from build123d import *

# Parameters (mm, degrees)
SKETCH1_R                      = 46
SKETCH1_R_2                    = 36.05
SKETCH1_R_3                    = 30
BOSS_EXTRUDE1_DEPTH            = 2
BOSS_EXTRUDE2_START            = -2
SKETCH1_3_R                    = 46
SKETCH1_3_R_2                  = 36.05
BOSS_EXTRUDE2_DEPTH            = 8
CBORE_FOR_M3_SHCS2_D           = 3.2
CBORE_FOR_M3_SHCS2_CBORE_D     = 6.5
CBORE_FOR_M3_SHCS2_CBORE_DEPTH = 3
SKETCH8_R                      = 3.25
SKETCH8_W                      = 10
SKETCH8_H                      = 6.5
CUT_EXTRUDE1_DEPTH             = 66.429351212
CIRPATTERN1_COUNT              = 4
SKETCH9_R                      = 1.55
CUT_EXTRUDE2_DEPTH             = 66.817930688
CUT_EXTRUDE3_START             = -2
SKETCH9_3_R                    = 1.55
CUT_EXTRUDE3_DEPTH             = 64.817930688
CIRPATTERN2_COUNT              = 4


with BuildPart() as part:
    # Sketch1 → Boss-Extrude1 (new body)
    # profile 1 of 2: a face of its own
    with BuildSketch(Plane(origin=(0, 0, 0), x_dir=(1, 0, 0), z_dir=(0, 1, 0))):
        with Locations(Location((0, 0, 0), (0, 0, 270))):
            Circle(SKETCH1_R)
        Circle(SKETCH1_R_2, mode=Mode.SUBTRACT)
    # profile 2 of 2: a face of its own
    with BuildSketch(Plane(origin=(0, 0, 0), x_dir=(1, 0, 0), z_dir=(0, 1, 0))):
        Circle(SKETCH1_R_2)
        with Locations(Location((0, 0, 0), (0, 0, 270))):
            Circle(SKETCH1_R_3, mode=Mode.SUBTRACT)
    extrude(amount=-BOSS_EXTRUDE1_DEPTH)

    # Sketch1<3> → Boss-Extrude2 (add)
    with BuildSketch(Plane(origin=(0, 0, 0), x_dir=(1, 0, 0), z_dir=(0, 1, 0)).offset(BOSS_EXTRUDE2_START)):
        with Locations(Location((0, 0, 0), (0, 0, 270))):
            Circle(SKETCH1_3_R)
        with Locations(Location((0, 0, 0), (0, 0, 270))):
            Circle(SKETCH1_3_R_2, mode=Mode.SUBTRACT)
    extrude(amount=-BOSS_EXTRUDE2_DEPTH)

    # CBORE for M3 SHCS2 (through all)
    with Locations(Plane(origin=(0, 0, 0), x_dir=(1, 0, 0), z_dir=(0, 1, 0))):
        with Locations((-42.5, 0)):
            cbore_for_m3_shcs2 = CounterBoreHole(CBORE_FOR_M3_SHCS2_D / 2, CBORE_FOR_M3_SHCS2_CBORE_D / 2, CBORE_FOR_M3_SHCS2_CBORE_DEPTH)

    # Sketch8 → Cut-Extrude1 (cut, through all)
    with BuildSketch(Plane(origin=(0, -3, 0), x_dir=(1, 0, 0), z_dir=(0, 1, 0))):
        with Locations((-42.5, 0)):
            Circle(SKETCH8_R)
        with Locations((-47.5, 0)):
            Rectangle(SKETCH8_W, SKETCH8_H)
    cut_extrude1 = extrude(amount=CUT_EXTRUDE1_DEPTH, mode=Mode.SUBTRACT)

    # CirPattern1: CBORE for M3 SHCS2, Cut-Extrude1 ×4 about axis
    cirpattern1_axis = Axis((0, 0, 0), (0, 1, 0))
    add([cbore_for_m3_shcs2.rotate(cirpattern1_axis, i * 360 / CIRPATTERN1_COUNT) for i in range(1, CIRPATTERN1_COUNT)], mode=Mode.SUBTRACT)
    add([cut_extrude1.rotate(cirpattern1_axis, i * 360 / CIRPATTERN1_COUNT) for i in range(1, CIRPATTERN1_COUNT)], mode=Mode.SUBTRACT)

    # Sketch9 → Cut-Extrude2 (cut, through all)
    with BuildSketch(Plane(origin=(0, 0, 0), x_dir=(1, 0, 0), z_dir=(0, 1, 0))):
        with Locations(Location((28.991378029, 28.991378029, 0), (0, 0, 270))):
            Circle(SKETCH9_R)
    cut_extrude2 = extrude(amount=-CUT_EXTRUDE2_DEPTH, mode=Mode.SUBTRACT)

    # Sketch9<3> → Cut-Extrude3 (cut, through all)
    with BuildSketch(Plane(origin=(0, 0, 0), x_dir=(1, 0, 0), z_dir=(0, 1, 0)).offset(CUT_EXTRUDE3_START)):
        Polygon((32.058604476, 29.813238878), (29.813238878, 32.058604476), (26.746012431, 31.236743626), (25.924151582, 28.169517179), (28.169517179, 25.924151582), (31.236743626, 26.746012431), align=None)
        with Locations(Location((28.991378029, 28.991378029, 0), (0, 0, 270))):
            Circle(SKETCH9_3_R, mode=Mode.SUBTRACT)
    cut_extrude3 = extrude(amount=-CUT_EXTRUDE3_DEPTH, mode=Mode.SUBTRACT)

    # CirPattern2: Cut-Extrude2, Cut-Extrude3 ×4 about axis
    cirpattern2_axis = Axis((0, 0, 0), (0, 1, 0))
    add([cut_extrude2.rotate(cirpattern2_axis, i * 360 / CIRPATTERN2_COUNT) for i in range(1, CIRPATTERN2_COUNT)], mode=Mode.SUBTRACT)
    add([cut_extrude3.rotate(cirpattern2_axis, i * 360 / CIRPATTERN2_COUNT) for i in range(1, CIRPATTERN2_COUNT)], mode=Mode.SUBTRACT)


solid = part.part
Geometry check sheet. Reference: the model listing, model coordinates, mm. A direction names the side the tool comes from. Give positions to 0.01 mm unless a question says otherwise; leave off trailing zeros. Write each loop counter-clockwise with the first axis right and the second up, starting at its lowest first coordinate (ties: lowest second). Pieces come first, ordered by that corner, then holes. Notation, with made-up numbers: M -12.75,-34 L 45.25,-34 A22 ccw 45.25,-28 Z; hole C 15.5,49 d6. An arc over 180 degrees is marked long. Answer as CSV lines item,"result". Start each with the question number.
Q1. Section check C-C, the plane y = -4.75. Give the number of separate pieces and of enclosed holes in the cut face, then the cut area to 3 significant figures.
Q2. Material ranges on L1, parallel to Z at x = -29, y = -8 (3 decimals); L2, parallel to Y at x = 24.5, z = 26; L3, parallel to Z at x = -22, y = -7.75, recorded low to high.
Q3. Section check D-D, the plane x = -13.5. Record the cut outline in (y, z), then the cut area to 3 significant figures.
Q4. Tool access check on faces 1 (the face through (-26.33, -5.94, -29.68)), 2 (the face through (3.25, -2, 44)), 3 (the face through (3.25, -2, -44)), 4 (the face through (-44, -2, -3.25)). Record the directions out of +Z, -Z, +X, -X, +Y, -Y that give a thin tool (end or side, any length) a straight path to the whole face; none if there is none.
Q5. Section check B-B, the plane z = 0. Record the cut outline in (x, y), then the cut area to 3 significant figures.
Q6. Release check for a two-part mould opening along Z. For faces 5 (the face through (-34, -10, 13)), 6 (the face through (41.32, -6.55, 1.08)) record: pulls with the +Z half, pulls with the -Z half, needs draft (parallel to the pull), parting line crosses it, or undercut.
Q7. Section check A-A, the plane x = 0. Record the cut outline in (y, z), then the cut area to 3 significant figures.
Q8. Go/stop test with flat-tipped pins: pin 1 (3.5 mm diameter, centred on x = 28.99, z = -28.99, fed in from -Y); pin 2 (2 mm diameter, centred on x = -2, y = -2.5, fed in from -Z); pin 3 (1 mm diameter, centred on x = -30.5, y = -4.5, fed in from -Z). Record where each tip stops, or that it passes through.
Geometry says:
1,separate pieces,"1"
1,enclosed holes,"9"
1,area,"2,430 mm^2"
2,L1,"-35.707 to -31.841, -26.147 to -21.415, 21.415 to 26.147, 31.841 to 35.707"
2,L2,"-2 to 0"
2,L3,"-40.4 to -28.56, 28.56 to 40.4"
3,outline,"M -10,-43.97 L 0,-43.97 L 0,-26.79 L -2,-26.79 L -2,-33.43 L -10,-33.43 Z; M -10,33.43 L -2,33.43 L -2,26.79 L 0,26.79 L 0,43.97 L -10,43.97 Z"
3,area,"237 mm^2"
4,face 1,"-Y"
4,face 2,"+Z, +Y"
4,face 3,"-Z, +Y"
4,face 4,"-X, +Y"
5,outline,"M -46,-10 L -44.1,-10 L -44.1,-3 L -46,-3 Z; M -40.9,-10 L -36.05,-10 L -36.05,-2 L -30,-2 L -30,0 L -39.25,0 L -39.25,-3 L -40.9,-3 Z; M 30,-2 L 36.05,-2 L 36.05,-10 L 40.9,-10 L 40.9,-3 L 39.25,-3 L 39.25,0 L 30,0 Z; M 44.1,-10 L 46,-10 L 46,-3 L 44.1,-3 Z"
5,area,"138 mm^2"
6,face 5,"needs draft"
6,face 6,"undercut"
7,outline,"M -10,-46 L -3,-46 L -3,-44.1 L -10,-44.1 Z; M -10,-40.9 L -3,-40.9 L -3,-39.25 L 0,-39.25 L 0,-30 L -2,-30 L -2,-36.05 L -10,-36.05 Z; M -10,36.05 L -2,36.05 L -2,30 L 0,30 L 0,39.25 L -3,39.25 L -3,40.9 L -10,40.9 Z; M -10,44.1 L -3,44.1 L -3,46 L -10,46 Z"
7,area,"138 mm^2"
8,pin 1,"y = -2"
8,pin 2,"z = -45.99"
8,pin 3,"z = -34.87"
